```python
from build123d import *

# Parameters (mm, degrees)
F0_W     = 229.329064
F0_H     = 29.990316
F1_DEPTH = 113.530092
F2_W     = 216.629066
F2_H     = 17.290316
F3_DEPTH = 26.342174
F5_W     = 229.329064
F5_H     = 29.990316
F6_DEPTH = 4.393091
F7_W     = 229.329064
F7_H     = 29.990316
F7_W_2   = 216.629066
F7_H_2   = 17.290316
F8_DEPTH = 455.099583


with BuildPart() as f1:
    # F0 (on Top) → F1 (new body)
    with BuildSketch(Plane.XY):
        Rectangle(F0_W, F0_H)
    extrude(amount=F1_DEPTH)

    # F2 (on face) → F3 (join)
    with BuildSketch(Plane.XY.offset(113.530092)):
        Rectangle(F2_W, F2_H)
    extrude(amount=F3_DEPTH)

    # F5 (on offset) → F6 (join)
    with BuildSketch(Plane.XY.offset(123.39519)):
        Rectangle(F5_W, F5_H)
    extrude(amount=F6_DEPTH)

    # F7 (on face) → F8 (join)
    with BuildSketch(Plane.XY.offset(139.872266)):
        Rectangle(F7_W, F7_H)
        Rectangle(F7_W_2, F7_H_2, mode=Mode.SUBTRACT)
        Rectangle(F7_W_2, F7_H_2)
    extrude(amount=F8_DEPTH)


solid = f1.part
```
CAD build for the part. Positions are in the model's coordinates, mm. A direction names the side the tool comes from. Give positions to 0.01 mm unless a question says otherwise; leave off trailing zeros. Order: outer loops, then holes, each group sorted by start corner. A loop starts at its lowest first (then second) coordinate and runs counter-clockwise, first axis right, second up.
(1) Flat gauge pins, fed straight in: pin 1 (6 mm diameter, centred on x = -47.5, z = 131, fed in from +Y); pin 2 (3.5 mm diameter, centred on y = 1.5, z = 136.5, fed in from -X); pin 3 (6 mm diameter, centred on x = 6, z = 132, fed in from -Y). Where does each tip first touch, or does it go through?
(2) Saw through at A-A, the plane x = -85. Give the cut face in (y, z), then the cut area to 3 significant figures.
(3) Drill centre lines: L1, parallel to Z at x = 75.5, y = 12.5; L2, parallel to X at y = -2, z = 130. Where is each one in solid material? Low to high.
(4) Tool access for faces 4 (the flat face through (108.315, 0, 134)), 5 (the flat face through (-2, -8.645, 118)), 6 (the flat face through (-108.315, 0, 118)): list every direction of +Z, -Z, +X, -X, +Y, -Y with a clear straight run to the whole face (end or side of a thin tool).
(5) Mould opens along Z. For faces 1 (the flat face through (-2, 0, 594.972)), 2 (the flat face through (-2, 10, 113.53)), 3 (the flat face through (-2, -14.995, 364)) say: released by +Z, released by -Z, zero draft, split by the parting line, or undercut.
Results found:
1. pin 1: stops at y = 8.65
1. pin 2: stops at x = -108.31
1. pin 3: stops at y = -8.65
2. outline: (-15, 0) - (15, 0) - (15, 113.53) - (8.65, 113.53) - (8.65, 123.4) - (15, 123.4) - (15, 127.79) - (8.65, 127.79) - (8.65, 139.87) - (15, 139.87) - (15, 594.97) - (-15, 594.97) - (-15, 139.87) - (-8.65, 139.87) - (-8.65, 127.79) - (-15, 127.79) - (-15, 123.4) - (-8.65, 123.4) - (-8.65, 113.53) - (-15, 113.53) - close
2. area: 17,600 mm2
3. L1: z = 0 to 113.53, 123.4 to 127.79, 139.87 to 594.97
3. L2: x = -108.31 to 108.31
4. face 4: +X, +Y, -Y
4. face 5: +X, -X, -Y
4. face 6: -X, +Y, -Y
5. face 1: released by +Z
5. face 2: undercut
5. face 3: zero draft
